from build123d import *

# Parameters (mm, degrees)
F0_R     = 76.2
F1_DEPTH = 6.35
F2_R     = 73.025
F3_DEPTH = 3.81
F4_R     = 2.712473
F4_R_2   = 3.175
F5_DEPTH = 6.351
F6_R     = 3.175
F6_R_2   = 2.966679
F7_DEPTH = 6.351


with BuildPart() as f1:
    # F0 (on Top) → F1 (new body)
    with BuildSketch(Plane.XY):
        Circle(F0_R)
    extrude(amount=F1_DEPTH)

    # F2 (on Top) → F3 (cut)
    with BuildSketch(Plane.XY):
        Circle(F2_R)
    extrude(amount=F3_DEPTH, mode=Mode.SUBTRACT)

    # F4 (on face) → F5 (cut, through all)
    with BuildSketch(Plane.XY.offset(6.35)):
        with Locations((-31.75, 0)):
            Circle(F4_R)
        with Locations((31.75, 0)):
            Circle(F4_R_2)
        Circle(F4_R_2)
    extrude(amount=-F5_DEPTH, mode=Mode.SUBTRACT)

    # F6 (on face) → F7 (cut, through all)
    with BuildSketch(Plane.XY.offset(6.35)):
        with Locations((0, 44.45)):
            Circle(F6_R)
        with Locations((0, -44.45)):
            Circle(F6_R_2)
    extrude(amount=-F7_DEPTH, mode=Mode.SUBTRACT)


solid = f1.part
Geometry: final body of the model. Coordinates: model frame, mm. A direction names the side the tool comes from. Round coordinates to 2 decimals unless told otherwise and drop trailing zeros. Loops run counter-clockwise (first coordinate to the right, second up) from the corner with the lowest first, then second, coordinate; pieces in that order, holes last. Notation, with made-up numbers: M 22.25,44 L 47.25,44 A18 ccw 47.25,75 Z; hole C -28,73.5 d11. An arc over 180 degrees is marked long. One line per question, with ' | ' between items.
(1) Cut plane D-D on x = -9. Return the cut outline in (y, z).
Check result:
outline: M -75.67,0 L -72.47,0 L -72.47,3.81 L 72.47,3.81 L 72.47,0 L 75.67,0 L 75.67,6.35 L -75.67,6.35 Z
(2) Access query for faces 1 (the flat face through (-1, -16, 6.35)), 2 (the cylindrical face through (69.653, 21.935, 1.878)). Directions: +Z, -Z, +X, -X, +Y, -Y. A direction counts if a zero-diameter tool reaches every point of the face in a straight line with its end or side. Return the directions, or none.
Check result:
face 1: +Z, +X, -X, +Y, -Y | face 2: -Z
(3) Cut plane B-B on y = -44.45. Return the cut outline in (x, z), plus the area to 3 significant figures.
Check result:
outline: M -61.89,0 L -57.94,0 L -57.94,3.81 L -2.97,3.81 L -2.97,6.35 L -61.89,6.35 Z; M 2.97,3.81 L 57.94,3.81 L 57.94,0 L 61.89,0 L 61.89,6.35 L 2.97,6.35 Z | area: 329 mm2
(4) Cut plane A-A on x = -31.75. Return the cut outline in (y, z).
Check result:
outline: M -69.27,0 L -65.76,0 L -65.76,3.81 L -2.71,3.81 L -2.71,6.35 L -69.27,6.35 Z; M 2.71,3.81 L 65.76,3.81 L 65.76,0 L 69.27,0 L 69.27,6.35 L 2.71,6.35 Z
(5) Material intervals for line 1 along Y through (x, z) = (0, 5.8) (3 decimals); line 2 along Z through (x, y) = (-43, -6); line 3 along Y through (x, z) = (23.5, 3), sorted ascending. Write a range as from..to.
Check result:
line 1: y = -76.2..-47.417, -41.483..-3.175, 3.175..41.275, 47.625..76.2 | line 2: z = 3.81..6.35 | line 3: y = -72.49..-69.14, 69.14..72.49
(6) Cut plane C-C on z = 5. Return the cut outline in (x, y) (3 decimals).
Check result:
outline: C 0,0 d152.4; hole C -31.75,0 d5.425; hole C 0,0 d6.35; hole C 0,44.45 d6.35; hole C 0,-44.45 d5.933; hole C 31.75,0 d6.35
(7) Pull-direction query (Y, two-part tool) for faces 3 (the cylindrical face through (-34.46, 0.12, 5.1)), 4 (the flat face through (39, -62, 0)), 5 (the flat face through (-1, -15, 3.81)), 6 (the cylindrical face through (-60.47, -46.367, 3.131)); classes: +Y half, -Y half, draft (parallel to the pull), parting line (faces both ways), or undercut.
Check result:
face 3: undercut | face 4: draft | face 5: undercut | face 6: parting line
(8) Contact query for flat-ended pins moving along their axis: P1, Ø8, axis at x = 56, y = -60.5, coming from the +Z side; P2, Ø3, axis at y = -31, z = 4, coming from the +X side; P3, Ø1, axis at x = 23.5, z = 2.5, coming from the +Y side; P4, Ø2, axis at x = -58.5, z = 5.5, coming from the -Y side. Output: stop coordinate, or through.
Check result:
P1: passes through | P2: stops at x = 70.26 | P3: stops at y = 72.65 | P4: stops at y = -50
